For this review, use the dimensioned drawing (mm, ordinates from the lowest corner) and the shaded views. Give positions to 0.01 mm unless a question says otherwise; leave off trailing zeros. Loops run counter-clockwise (first coordinate to the right, second up) from the corner with the lowest first, then second, coordinate; pieces in that order, holes last. Notation, with made-up numbers: M 10.5,20.25 L 44.5,20.25 A14 ccw 44.5,27.25 Z; hole C -7,86 d2. An arc over 180 degrees is marked long. Use CSV: the item, a comma, the result in double quotes.
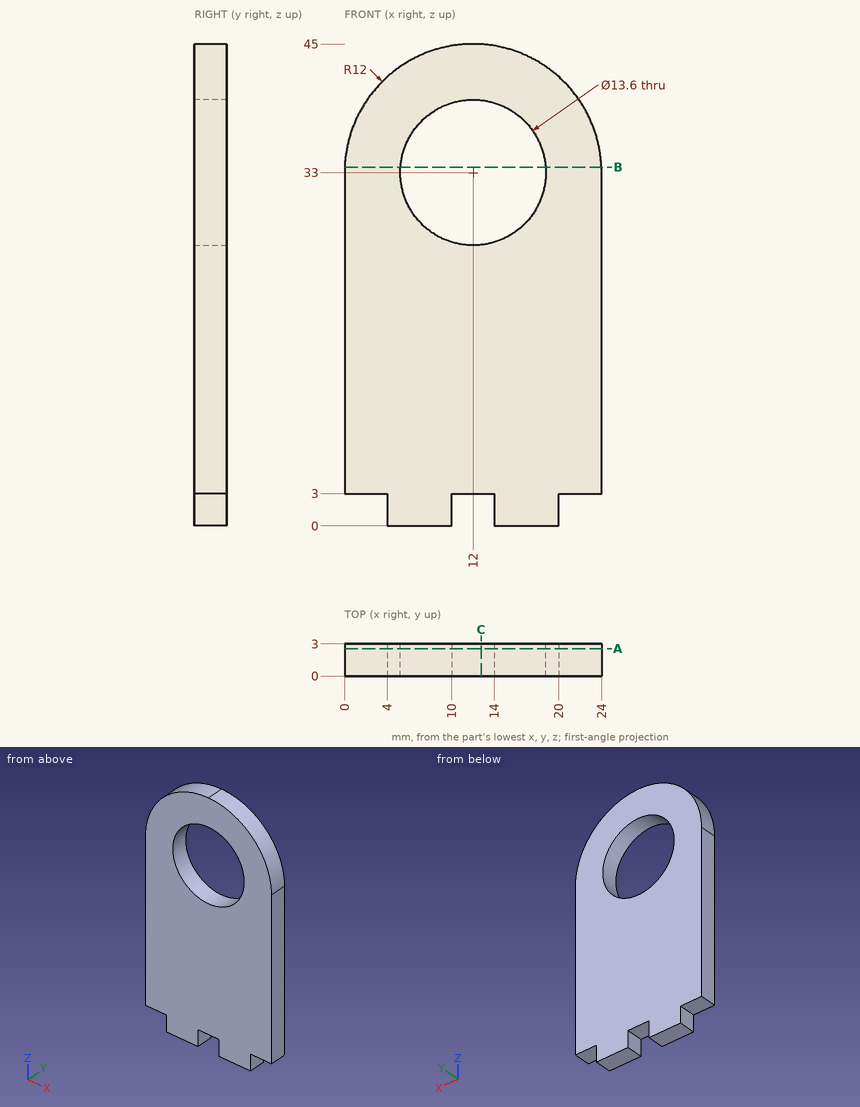
(1) Wall thickness on line 1 along X through (y, z) = (1.15, 33); line 2 along Z through (x, y) = (7.75, 1.35); line 3 along X through (y, z) = (2.8, 27.5): over which ranges is each line inside the solid? List them lowest first. Write a range as [from, to].
A:
line 1,"[0, 5.2], [18.8, 24]"
line 2,"[0, 27.69], [38.31, 44.22]"
line 3,"[0, 8], [16, 24]"
(2) Clearance check with flat-ended pins moving along their axes: P1, Ø8, axis at x = 12, z = 33, coming from the +Y side; P2, Ø0.9, axis at y = 2, z = 1.5, coming from the +X side; P3, Ø1.5, axis at x = 2, y = 2, coming from the -Z side. State where each tip first meets the part, or that it passes through.
A:
P1,"through"
P2,"x = 20"
P3,"z = 3"
(3) We need section A-A on y = 2.55. State the section outline as (x, z) points.
A:
outline,"M 0,3 L 4,3 L 4,0 L 10,0 L 10,3 L 14,3 L 14,0 L 20,0 L 20,3 L 24,3 L 24,33 A12 ccw 12,45 A12 ccw 0,33 Z; hole C 12,33 d13.6"
(4) We need section B-B on z = 33.5. State the section outline as (x, y) points, then the cut area to 3 significant figures.
A:
outline,"M 0.01,0 L 5.22,0 L 5.22,3 L 0.01,3 Z; M 18.78,0 L 23.99,0 L 23.99,3 L 18.78,3 Z"
area,"31.2 mm²"
(5) We need section C-C on x = 12.75. State the section outline as (y, z) points.
A:
outline,"M 0,3 L 3,3 L 3,26.24 L 0,26.24 Z; M 0,39.76 L 3,39.76 L 3,44.98 L 0,44.98 Z"
